from build123d import *

# Parameters (mm, degrees)
EXTRUDE_1_DEPTH         = 2000
EXTRUDE_2_DEPTH         = 5
HOLE_WIZARD_16_0_16_1_D = 16


with BuildPart() as part:
    # Model → 凸台-拉伸1 (new body)
    with BuildSketch(Plane.XY):
        with BuildLine():
            Line((55, -147), (6, -147))
            Line((6, -147), (6, -150))
            Line((6, -150), (0, -150))
            Line((0, -150), (0, 0))
            Line((0, 0), (150, 0))
            Line((150, 0), (150, -6))
            Line((150, -6), (147, -6))
            Line((147, -6), (147, -55))
            Line((147, -55), (150, -58))
            Line((150, -58), (150, -65))
            Line((150, -65), (142, -65))
            Line((142, -65), (142, -6))
            Line((142, -6), (9, -6))
            ThreePointArc((9, -6), (6.878679656, -6.878679656), (6, -9))
            Line((6, -9), (6, -142))
            Line((6, -142), (65, -142))
            Line((65, -142), (65, -150))
            Line((65, -150), (58, -150))
            Line((58, -150), (55, -147))
        make_face()
    extrude(amount=EXTRUDE_1_DEPTH)

    # 草图2 → 凸台-拉伸2 (add)
    with BuildSketch(Plane.XY.offset(2000)):
        Polygon((65, -142), (65, -65), (142, -65), (142, -6), (6, -6), (6, -142), align=None)
    extrude_2 = extrude(amount=-EXTRUDE_2_DEPTH)

    # 镜向1: 凸台-拉伸2 across plane
    add(extrude_2.mirror(Plane.XY.offset(1000)))

    # Ø16.0 (16) 直径孔1 (through all)
    with Locations(Plane.XY.offset(2000)):
        with Locations((100, -32.5), (32.5, -100)):
            Hole(HOLE_WIZARD_16_0_16_1_D / 2)


solid = part.part
Source: CAD feature listing. Evaluate the final solid. Frame: model axes, mm. A direction names the side the tool comes from. Round coordinates to 2 decimals unless told otherwise and drop trailing zeros. Write each loop counter-clockwise with the first axis right and the second up, starting at its lowest first coordinate (ties: lowest second). Pieces come first, ordered by that corner, then holes. Notation, with made-up numbers: M 24.25,-20 L 65.25,-20 A28 ccw 65.25,13 Z; hole C -22.5,-36 d2. An arc over 180 degrees is marked long. One line per item, written item: value. Start each with the question number.
Item 1: Set-up query: faces 1 (the flat face through (31, -147, 986)), 2 (the flat face through (145, -65, 995)), 3 (the flat face through (147, -30, 986)), 4 (the flat face through (58, -58, 5)). Return all of +Z, -Z, +X, -X, +Y, -Y with unobstructed straight access to the full face (end or side cutting, diameter ignored); none if empty.
Item 2: Section query A-A (z = 590.5). Return the cut outline in (x, y), plus the area to 3 significant figures.
Item 3: Mould query, pull axis Z, two halves, no side actions, for faces 5 (the flat face through (57, -57, 0)), 6 (the flat face through (57, -57, 2000)), 7 (the flat face through (142, -36, 986)). Classes: pulls with the +Z half, pulls with the -Z half, needs draft (parallel to the pull), parting line crosses it, or undercut.
Item 4: Ray query, L1, parallel to Z at x = 111, y = -21; L2, parallel to Y at x = 32, z = 1997; L3, parallel to Y at x = 100, z = 2. Return the intervals inside material, ascending. Write a range as from..to.
Item 5: Pin query (flat end, axial travel): pin 1 (1.5 mm diameter, centred on y = -108, z = 1315, fed in from +X); pin 2 (0.9 mm diameter, centred on x = 148, z = 613, fed in from -Y); pin 3 (3.5 mm diameter, centred on y = -149, z = 526, fed in from +X). Return the tip coordinate at first contact, or that it passes through.
Result set:
1. face 1: +Z, -Z, -Y
1. face 2: +Z, -Z, +X, -Y
1. face 3: +Z, -Z, +X
1. face 4: none
2. outline: M 0,-150 L 6,-150 L 6,-147 L 55,-147 L 58,-150 L 65,-150 L 65,-142 L 6,-142 L 6,-9 A3 cw 9,-6 L 142,-6 L 142,-65 L 150,-65 L 150,-58 L 147,-55 L 147,-6 L 150,-6 L 150,0 L 0,0 Z
2. area: 2,410 mm²
3. face 5: pulls with the -Z half
3. face 6: pulls with the +Z half
3. face 7: undercut
4. L1: z = 0..5, 1995..2000
4. L2: y = -147..-107.98, -92.02..0
4. L3: y = -65..-40.5, -24.5..0
5. pin 1: stops at x = 6
5. pin 2: stops at y = -65
5. pin 3: stops at x = 65
